Build history of the part. All positions in model axes, mm. Face numbers are marked on the shaded views. Round coordinates to 2 decimals unless told otherwise and drop trailing zeros. Loops run counter-clockwise (first coordinate to the right, second up) from the corner with the lowest first, then second, coordinate; pieces in that order, holes last.
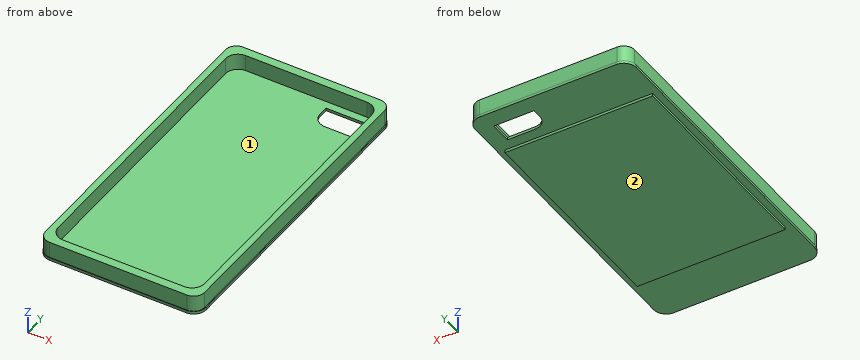
from build123d import *

# Parameters (mm, degrees)
F1_W     = 68.8515231013
F1_H     = 100.0347808003
F2_DEPTH = 1.27
F3_DEPTH = 7.62
F4_DEPTH = 2.54


with BuildPart() as f2:
    # F1 (on Top) → F2 (new body)
    with BuildSketch(Plane.XY):
        with BuildLine():
            ThreePointArc((-37.5236049294, -67.3895406203), (-35.8125227451, -71.520458436), (-31.6816049294, -73.2315406203))
            Line((-31.6816049294, -73.2315406203), (31.6816049294, -73.2315406203))
            ThreePointArc((31.6816049294, -73.2315406203), (35.8125227451, -71.520458436), (37.5236049294, -67.3895406203))
            Line((37.5236049294, -67.3895406203), (37.5236049294, 67.3895406203))
            ThreePointArc((37.5236049294, 67.3895406203), (35.8125227451, 71.520458436), (31.6816049294, 73.2315406203))
            Line((31.6816049294, 73.2315406203), (-31.6816049294, 73.2315406203))
            ThreePointArc((-31.6816049294, 73.2315406203), (-35.8125227451, 71.520458436), (-37.5236049294, 67.3895406203))
            Line((-37.5236049294, 67.3895406203), (-37.5236049294, -67.3895406203))
        make_face()
        Rectangle(F1_W, F1_H, mode=Mode.SUBTRACT)
        with BuildLine():
            Line((11.3956173882, 65.3541386127), (30.0525762141, 65.3541386127))
            Line((30.0525762141, 65.3541386127), (30.0525762141, 55.0315789878))
            Line((30.0525762141, 55.0315789878), (17.2376173882, 55.0315789878))
            ThreePointArc((17.2376173882, 55.0315789878), (13.1066995725, 56.7426611721), (11.3956173882, 60.8735789878))
            Line((11.3956173882, 60.8735789878), (11.3956173882, 65.3541386127))
        make_face(mode=Mode.SUBTRACT)
    extrude(amount=-F2_DEPTH)

    # F0 (on Top) → F3 (join)
    with BuildSketch(Plane.XY):
        with BuildLine():
            Line((31.9594252241, 72.9894563556), (-31.9594252241, 72.9894563556))
            ThreePointArc((-31.9594252241, 72.9894563556), (-35.5515276725, 71.501558804), (-37.0394252241, 67.9094563556))
            Line((-37.0394252241, 67.9094563556), (-37.0394252241, -67.9094563556))
            ThreePointArc((-37.0394252241, -67.9094563556), (-35.5515276725, -71.501558804), (-31.9594252241, -72.9894563556))
            Line((-31.9594252241, -72.9894563556), (31.9594252241, -72.9894563556))
            ThreePointArc((31.9594252241, -72.9894563556), (35.5515276725, -71.501558804), (37.0394252241, -67.9094563556))
            Line((37.0394252241, -67.9094563556), (37.0394252241, 67.9094563556))
            ThreePointArc((37.0394252241, 67.9094563556), (35.5515276725, 71.501558804), (31.9594252241, 72.9894563556))
        make_face()
        with BuildLine():
            Line((-28.2269942241, 68.9697414637), (28.2269942241, 68.9697414637))
            ThreePointArc((28.2269942241, 68.9697414637), (32.3579120398, 67.2586592794), (34.0689942241, 63.1277414637))
            Line((34.0689942241, 63.1277414637), (34.0689942241, -63.1277414637))
            ThreePointArc((34.0689942241, -63.1277414637), (32.3579120398, -67.2586592794), (28.2269942241, -68.9697414637))
            Line((28.2269942241, -68.9697414637), (-28.2269942241, -68.9697414637))
            ThreePointArc((-28.2269942241, -68.9697414637), (-32.3579120398, -67.2586592794), (-34.0689942241, -63.1277414637))
            Line((-34.0689942241, -63.1277414637), (-34.0689942241, 63.1277414637))
            ThreePointArc((-34.0689942241, 63.1277414637), (-32.3579120398, 67.2586592794), (-28.2269942241, 68.9697414637))
        make_face(mode=Mode.SUBTRACT)
    extrude(amount=F3_DEPTH)

    # F1 (on Top) → F4 (join)
    with BuildSketch(Plane.XY):
        Rectangle(F1_W, F1_H)
    extrude(amount=-F4_DEPTH)


solid = f2.part
(1) Slice it at C-C on y = 57. List the corners of the cut face in (x, z).
Responses:
outline: (-37.52, -1.27) - (12.86, -1.27) - (12.86, 0) - (-34.07, 0) - (-34.07, 7.62) - (-37.04, 7.62) - (-37.04, 0) - (-37.52, 0) - close; (30.05, -1.27) - (37.52, -1.27) - (37.52, 0) - (37.04, 0) - (37.04, 7.62) - (34.07, 7.62) - (34.07, 0) - (30.05, 0) - close
(2) Slice it at D-D on x = -23. List the corners of the cut face in (y, z), plus the area to 3 significant figures.
Responses:
outline: (-73.23, -1.27) - (-50.02, -1.27) - (-50.02, -2.54) - (50.02, -2.54) - (50.02, -1.27) - (73.23, -1.27) - (73.23, 0) - (72.99, 0) - (72.99, 7.62) - (68.97, 7.62) - (68.97, 0) - (-68.97, 0) - (-68.97, 7.62) - (-72.99, 7.62) - (-72.99, 0) - (-73.23, 0) - close
area: 374 mm2
(3) Slice it at A-A on x = 25. List the corners of the cut face in (y, z), plus the area to 3 significant figures.
Responses:
outline: (-73.23, -1.27) - (-50.02, -1.27) - (-50.02, -2.54) - (50.02, -2.54) - (50.02, -1.27) - (55.03, -1.27) - (55.03, 0) - (-68.97, 0) - (-68.97, 7.62) - (-72.99, 7.62) - (-72.99, 0) - (-73.23, 0) - close; (65.35, -1.27) - (73.23, -1.27) - (73.23, 0) - (72.99, 0) - (72.99, 7.62) - (68.97, 7.62) - (68.97, 0) - (65.35, 0) - close
area: 361 mm2
(4) Pull direction Y, two halves, no side cores. Call the marked faces 1 and 2: +Y half, -Y half, draft (parallel to the pull), parting line (faces both ways), or undercut.
Responses:
face 1: undercut
face 2: draft
(5) Pin check, flat tips, straight feed: P1, Ø6, axis at x = 13, z = 5.5, coming from the +Y side; P2, Ø1, axis at y = -49, z = 2, coming from the -X side; P3, Ø4, axis at y = 2.5, z = 4, coming from the +X side; P4, Ø5, axis at y = 4.5, z = 1.5, coming from the -X side. Stop position of each tip, or through.
Responses:
P1: stops at y = 72.99
P2: stops at x = -37.04
P3: stops at x = 37.04
P4: stops at x = -37.52
(6) Probe line 1 (X direction, y = 28, z = 3.25); line 2 (Y direction, x = -5, z = 6); line 3 (Z direction, x = -1, y = 38). List the from-to ranges inside material, lowest first.
Responses:
line 1: x = -37.04 to -34.07, 34.07 to 37.04
line 2: y = -72.99 to -68.97, 68.97 to 72.99
line 3: z = -2.54 to 0
(7) Slice it at B-B on z = 3.5. List the corners of the cut face in (x, y).
Responses:
outline: (-37.04, -67.91) arc R5.08 ccw to (-31.96, -72.99) - (31.96, -72.99) arc R5.08 ccw to (37.04, -67.91) - (37.04, 67.91) arc R5.08 ccw to (31.96, 72.99) - (-31.96, 72.99) arc R5.08 ccw to (-37.04, 67.91) - close; hole (-34.07, -63.13) arc R5.84 ccw to (-28.23, -68.97) - (28.23, -68.97) arc R5.84 ccw to (34.07, -63.13) - (34.07, 63.13) arc R5.84 ccw to (28.23, 68.97) - (-28.23, 68.97) arc R5.84 ccw to (-34.07, 63.13) - close
